Could you check a few things on this model? Use its own coordinates, in mm. Face numbers are marked on the shaded views. A direction names the side the tool comes from. Coordinates: 2 decimals unless noted, no trailing zeros. Loops run counter-clockwise (first coordinate to the right, second up) from the corner with the lowest first, then second, coordinate; pieces in that order, holes last.
from build123d import *

# Parameters (mm, degrees)
SKETCH2_R           = 10
SKETCH2_R_2         = 2.5
BOSS_EXTRUDE1_DEPTH = 5


with BuildPart() as part:
    # Sketch2 → Boss-Extrude1 (new body)
    with BuildSketch(Plane.XY):
        with BuildLine():
            Line((0, 0), (70, 0))
            ThreePointArc((70, 0), (80, 10), (70, 20))
            Line((70, 20), (30, 20))
            Line((30, 20), (30, 80))
            ThreePointArc((30, 80), (15, 95), (0, 80))
            Line((0, 80), (0, 0))
        make_face()
        with Locations((15, 80)):
            Circle(SKETCH2_R, mode=Mode.SUBTRACT)
        with Locations((15, 20)):
            Circle(SKETCH2_R_2, mode=Mode.SUBTRACT)
        with Locations((15, 40)):
            Circle(SKETCH2_R_2, mode=Mode.SUBTRACT)
        with Locations((55, 12)):
            Circle(SKETCH2_R_2, mode=Mode.SUBTRACT)
    extrude(amount=BOSS_EXTRUDE1_DEPTH)


solid = part.part
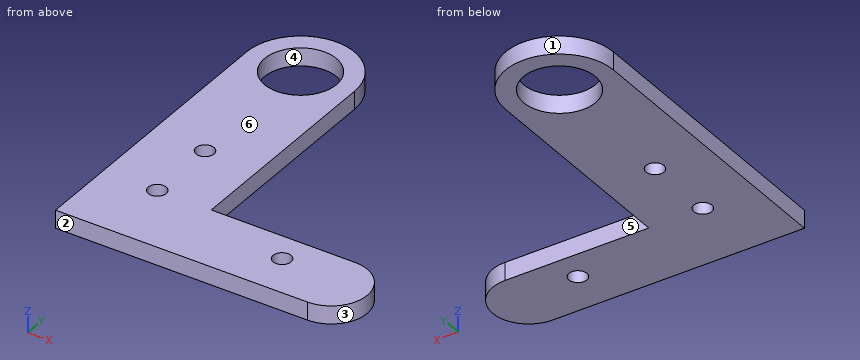
1) Imagine slicing it at B-B on x = 55. List the corners of the cut face in (y, z) for me, plus the area to 3 significant figures.
2) We'd pull the mould along X, two halves only. Please class the marked faces 1, 2, 3 and 4: released by +X, released by -X, zero draft, split by the parting line, or undercut.
3) For the marked faces 5 and 6, which set-ups out of +Z, -Z, +X, -X, +Y, -Y let a thin tool reach every point of the face, with its end or its side?
4) Will these pins go through, and if not, where does the flat tip stop? pin 1 (2.5 mm diameter, centred on y = 59, z = 1.5, fed in from +X); pin 2 (4 mm diameter, centred on x = 15, y = 40, fed in from +Z); pin 3 (8 mm diameter, centred on x = 15, y = 20, fed in from +Z); pin 4 (3 mm diameter, centred on x = 20, z = 4, fed in from +Y).
5) Imagine slicing it at D-D on y = 27.5. List the corners of the cut face in (x, z) for me, plus the area to 3 significant figures.
6) If I drill on L1, parallel to X at y = 66, z = 2.75; L2, parallel to Y at x = 45.5, z = 1.95; L3, parallel to X at y = 83, z = 3.15, over which ranges is the centre line in solid material (lowest first)?
7) Imagine slicing it at C-C on z = 3.7. List the corners of the cut face in (x, y) for me.
8) Imagine slicing it at A-A on y = 40. List the corners of the cut face in (x, z) for me, plus the area to 3 significant figures.
Solved:
1. outline: (0, 0) - (9.5, 0) - (9.5, 5) - (0, 5) - close; (14.5, 0) - (20, 0) - (20, 5) - (14.5, 5) - close
1. area: 75.0 mm2
2. face 1: split by the parting line
2. face 2: zero draft
2. face 3: released by +X
2. face 4: undercut
3. face 5: +Z, -Z, +X, +Y
3. face 6: +Z, +X, -X, +Y, -Y
4. pin 1: stops at x = 30
4. pin 2: passes through
4. pin 3: stops at z = 5
4. pin 4: stops at y = 94.59
5. outline: (0, 0) - (30, 0) - (30, 5) - (0, 5) - close
5. area: 150 mm2
6. L1: x = 0 to 30
6. L2: y = 0 to 20
6. L3: x = 0.3 to 5.46, 24.54 to 29.7
7. outline: (0, 0) - (70, 0) arc R10 ccw to (70, 20) - (30, 20) - (30, 80) arc R15 ccw to (0, 80) - close; hole circle Ø20 at (15, 80); hole circle Ø5 at (15, 20); hole circle Ø5 at (15, 40); hole circle Ø5 at (55, 12)
8. outline: (0, 0) - (12.5, 0) - (12.5, 5) - (0, 5) - close; (17.5, 0) - (30, 0) - (30, 5) - (17.5, 5) - close
8. area: 125 mm2
